from build123d import *

# Parameters (mm, degrees)
BOSS_EXTRUDE1_DEPTH = 2
SKETCH2_R           = 2.5
BOSS_EXTRUDE2_DEPTH = 9


with BuildPart() as part:
    # Sketch1 → Boss-Extrude1 (new, symmetric)
    with BuildSketch(Plane.XY):
        Polygon((5, 0), (2.5, 4.330127019), (-2.5, 4.330127019), (-5, 0), (-2.5, -4.330127019), (2.5, -4.330127019), align=None)
    extrude(amount=BOSS_EXTRUDE1_DEPTH, both=True)

    # Sketch2 → Boss-Extrude2 (add)
    with BuildSketch(Plane.XY.offset(2)):
        Circle(SKETCH2_R)
    extrude(amount=BOSS_EXTRUDE2_DEPTH)


solid = part.part
Part model, mm, in its own coordinate system. A direction names the side the tool comes from. Round coordinates to 2 decimals unless told otherwise and drop trailing zeros. Loops run counter-clockwise (first coordinate to the right, second up) from the corner with the lowest first, then second, coordinate; pieces in that order, holes last. Notation, with made-up numbers: (-9, -24.5) - (22, -24.5) arc R17 ccw to (22, -3.5) - close; hole circle Ø2 at (15.25, 50.25). An arc over 180 degrees is marked (long way). Answer as a JSON object with one key per item and string values.
Item 1: Band-saw the part on C-C on z = 9.5. List the corners of the cut face in (x, y).
Output:
{"outline": "circle Ø5 at (0, 0)"}
Item 2: Pin check, flat tips, straight feed: pin 1 (1.5 mm diameter, centred on x = -0.5, z = 7.5, fed in from +Y); pin 2 (3 mm diameter, centred on y = -2.5, z = 6, fed in from +X); pin 3 (6 mm diameter, centred on x = -3, z = 1, fed in from +Y); pin 4 (2 mm diameter, centred on y = 0, z = 4.5, fed in from +X). Stop position of each tip, or through.
Output:
{"pin 1": "y = 2.5", "pin 2": "x = 2.29", "pin 3": "y = 4.33", "pin 4": "x = 2.5"}
Item 3: Band-saw the part on D-D on y = -3. List the corners of the cut face in (x, z), plus the area to 3 significant figures.
Output:
{"outline": "(-3.27, -2) - (3.27, -2) - (3.27, 2) - (-3.27, 2) - close", "area": "26.1 mm2"}
Item 4: Band-saw the part on B-B on y = 1. List the corners of the cut face in (x, z), plus the area to 3 significant figures.
Output:
{"outline": "(-4.42, -2) - (4.42, -2) - (4.42, 2) - (2.29, 2) - (2.29, 11) - (-2.29, 11) - (-2.29, 2) - (-4.42, 2) - close", "area": "76.6 mm2"}
Item 5: Wall check: L1, parallel to Z at x = 2.25, y = -4; L2, parallel to X at y = -0.25, z = 9; L3, parallel to X at y = 1.25, z = 3.5. Give the ranges that are in metal, low to high.
Output:
{"L1": "-2 to 2", "L2": "-2.49 to 2.49", "L3": "-2.17 to 2.17"}
Item 6: Band-saw the part on A-A on x = 0. List the corners of the cut face in (y, z).
Output:
{"outline": "(-4.33, -2) - (4.33, -2) - (4.33, 2) - (2.5, 2) - (2.5, 11) - (-2.5, 11) - (-2.5, 2) - (-4.33, 2) - close"}
Item 7: Tool access for faces 1 (the face through (0, -4.33, 0)), 2 (the face through (-0.54, -2.44, 6.44)): list every direction of +Z, -Z, +X, -X, +Y, -Y with a clear straight run to the whole face (end or side of a thin tool).
Output:
{"face 1": "+Z, -Z, +X, -X, -Y", "face 2": "+Z"}
